from build123d import *

# Parameters (mm, degrees)
F0_W     = 25.4
F0_H     = 25.4
F0_W_2   = 20.32
F0_H_2   = 20.32
F1_DEPTH = 2.54
F2_DEPTH = 22.86
F3_W     = 10.16
F3_H     = 2.54
F4_DEPTH = 2.54
F6_DEPTH = 10.16
F7_W     = 2.54
F7_H     = 1.1816583352
F8_DEPTH = 2.54


with BuildPart() as f1:
    # F0 (on Top) → F1 (new body)
    with BuildSketch(Plane.XY):
        with Locations((0.373007264, -0.8804095839)):
            Rectangle(F0_W, F0_H)
        with Locations((0.373007264, -0.8804095839)):
            Rectangle(F0_W_2, F0_H_2, mode=Mode.SUBTRACT)
        with Locations((0.373007264, -0.8804095839)):
            Rectangle(F0_W_2, F0_H_2)
    extrude(amount=F1_DEPTH)

    # F0 (on Top) → F2 (join)
    with BuildSketch(Plane.XY):
        with Locations((0.373007264, -0.8804095839)):
            Rectangle(F0_W, F0_H)
        with Locations((0.373007264, -0.8804095839)):
            Rectangle(F0_W_2, F0_H_2, mode=Mode.SUBTRACT)
    extrude(amount=F2_DEPTH)

    # F3 (on face) → F4 (cut)
    with BuildSketch(Plane.XZ.offset(13.5804095839)):
        with Locations((0.373007264, 21.59)):
            Rectangle(F3_W, F3_H)
    extrude(amount=-F4_DEPTH, mode=Mode.SUBTRACT)

    # F5 (on face) → F6 (join)
    with BuildSketch(Plane.YZ.offset(-4.706992736)):
        with BuildLine():
            ThreePointArc((-11.9946550142, 21.5179765421), (-11.742671758, 21.7606545967), (-11.6500095839, 22.098))
            ThreePointArc((-11.6500095839, 22.098), (-12.6630783121, 22.6563483931), (-12.5941432245, 21.5016583352))
            ThreePointArc((-12.5941432245, 21.5016583352), (-12.29244, 21.4378445228), (-11.9946550142, 21.5179765421))
        make_face()
        with BuildLine():
            ThreePointArc((-11.9946550142, 21.5179765421), (-12.29244, 21.4378445228), (-12.5941432245, 21.5016583352))
            Line((-12.5941432245, 21.5016583352), (-12.5941432245, 21.4954577436))
            Line((-12.5941432245, 21.4954577436), (-12.5941432245, 20.32))
            Line((-12.5941432245, 20.32), (-11.9946550142, 20.32))
            Line((-11.9946550142, 20.32), (-11.9946550142, 21.4800578359))
            Line((-11.9946550142, 21.4800578359), (-11.9946550142, 21.5179765421))
        make_face()
    extrude(amount=F6_DEPTH)

    # F7 (on face) → F8 (cut)
    with BuildSketch(Plane.XZ.offset(12.5941432245)):
        with Locations((-2.420992736, 20.9108291676)):
            Rectangle(F7_W, F7_H)
        with Locations((3.167007264, 20.9108291676)):
            Rectangle(F7_W, F7_H)
    extrude(amount=-F8_DEPTH, mode=Mode.SUBTRACT)


solid = f1.part
Verification items for the finished model (mm, model axes). A direction names the side the tool comes from. Coordinates: 2 decimals unless noted, no trailing zeros. Order: outer loops, then holes, each group sorted by start corner. A loop starts at its lowest first (then second) coordinate and runs counter-clockwise, first axis right, second up. Notation, with made-up numbers: (85, -28) -> (132, -28) arc R18 ccw to (132, -8) -> close; hole circle Ø11 at (-13.75, 1). An arc over 180 degrees is marked (long way). Use CSV: the item, a comma, the result in double quotes. Start each with the question number.
Q1. Tool access check on faces 5 (the flat face through (0, -11.04, 13)), 6 (the flat face through (-4.707, -13, 21)), 7 (the flat face through (5, -12.594, 21)), 8 (the flat face through (0, -13.58, 11)). Record the directions out of +Z, -Z, +X, -X, +Y, -Y that give a thin tool (end or side, any length) a straight path to the whole face; none if there is none.
Q2. Section check B-B, the plane z = 8.75. Record the cut outline in (x, y), and give its area (3 significant figures).
Q3. Section check C-C, the plane x = 7.5. Record the cut outline in (y, z), and give its area (3 significant figures).
Q4. Thickness scan on line 1 along Y through (x, z) = (6.5, 7); line 2 along X through (y, z) = (8, 17.75); line 3 along Z through (x, y) = (8.25, 8.25). Record the ranges inside material, lowest first.
Q5. Section check D-D, the plane y = -7.5. Record the cut outline in (x, z), and give its area (3 significant figures).
Q6. Draft check along Y on faces 1 (the flat face through (-3, 10, 22.86)), 2 (the flat face through (-4, -12.594, 21)), 3 (the flat face through (0, 9.28, 13)), 4 (the flat face through (5.453, -13, 21)). Enter one of: +Y half, -Y half, draft (parallel to the pull), parting line (faces both ways), or undercut.
Q7. Depth check by flat-ended pin: P1, Ø0.8, axis at x = 5, z = 21, coming from the -Y side; P2, Ø8, axis at x = -3.5, y = -1, coming from the +Z side. Enter the tip coordinate at first touch or a pass-through.
Returned:
1,face 5,"+Z"
1,face 6,"none"
1,face 7,"-Y"
1,face 8,"+Z, -Z, +X, -X, -Y"
2,outline,"(-12.33, -13.58) -> (13.07, -13.58) -> (13.07, 11.82) -> (-12.33, 11.82) -> close; hole (-9.79, -11.04) -> (10.53, -11.04) -> (10.53, 9.28) -> (-9.79, 9.28) -> close"
2,area,"232 mm^2"
3,outline,"(-13.58, 0) -> (11.82, 0) -> (11.82, 22.86) -> (9.28, 22.86) -> (9.28, 2.54) -> (-11.04, 2.54) -> (-11.04, 22.86) -> (-13.58, 22.86) -> close"
3,area,"168 mm^2"
4,line 1,"y = -13.58 to -11.04, 9.28 to 11.82"
4,line 2,"x = -12.33 to -9.79, 10.53 to 13.07"
4,line 3,"z = 0 to 2.54"
5,outline,"(-12.33, 0) -> (13.07, 0) -> (13.07, 22.86) -> (10.53, 22.86) -> (10.53, 2.54) -> (-9.79, 2.54) -> (-9.79, 22.86) -> (-12.33, 22.86) -> close"
5,area,"168 mm^2"
6,face 1,"draft"
6,face 2,"-Y half"
6,face 3,"undercut"
6,face 4,"undercut"
7,P1,"stops at y = -12.59"
7,P2,"stops at z = 2.54"
